Read the model definition and answer for the solid it produces. Units are mm, in the model's axes. Face numbers are marked on the shaded views. A direction names the side the tool comes from. Coordinates: 2 decimals unless noted, no trailing zeros. Write each loop counter-clockwise with the first axis right and the second up, starting at its lowest first coordinate (ties: lowest second). Pieces come first, ordered by that corner, then holes.
(1) Determine the mould class of the marked faces 3, 4 and 5 for opening direction Y: pulls with the +Y half, pulls with the -Y half, needs draft (parallel to the pull), parting line crosses it, or undercut.
(2) The part is cut by section A-A, the plane z = -10. Determine the outline of the cut face in (x, y), and give its area (3 significant figures).
(3) The part is cut by section D-D, the plane z = 0. Determine the outline of the cut face in (x, y), and give its area (3 significant figures).
(4) The part is cut by section B-B, the plane y = 0. Determine the outline of the cut face in (x, z).
(5) The part is cut by section C-C, the plane x = 0. Determine the outline of the cut face in (y, z).
(6) Straight lines are drawn through the part: line 1 along X through (y, z) = (-16.5, 2); line 2 along Z through (x, y) = (-2, -8); line 3 along Y through (x, z) = (-24, 0). For each, find the intervals that lie inside material, in ascending order.
(7) Given pin 1 (24 mm diameter, centred on x = -2, y = 2, fed in from +Z); pin 2 (1.8 mm diameter, centred on x = 17.5, y = -6.5, fed in from +Z), each flat-ended and moving along its own axis, determine where each tip first touches the part or whether it passes through.
(8) Which of the six approach directions +Z, -Z, +X, -X, +Y, -Y give full straight-line access (tool end or side, diameter ignored) to the marked faces 1 and 2?
```python
from build123d import *

# Parameters (mm, degrees)
SKETCH1_R           = 7.5
BOSS_EXTRUDE1_DEPTH = 29
CUT_EXTRUDE1_DEPTH  = 68.505555327
SKETCH3_R           = 7
CUT_EXTRUDE2_DEPTH  = 85.917607126
CUT_EXTRUDE3_DEPTH  = 68.505555438


with BuildPart() as part:
    # Sketch1 → Boss-Extrude1 (new, symmetric)
    with BuildSketch(Plane(origin=(0, 0, 0), x_dir=(0, 0, -1), z_dir=(1, 0, 0))):
        with BuildLine():
            Line((-31, 5), (-31, -19))
            Line((-31, -19), (31, -19))
            Line((31, -19), (46, -10.339745962))
            Line((46, -10.339745962), (46, 12.339745962))
            Line((46, 12.339745962), (31, 21))
            Line((31, 21), (5.66060556, 21))
            ThreePointArc((5.66060556, 21), (-14.33939444, 16.82575695), (-31, 5))
        make_face()
        with Locations(Location((0, 0, 0), (0, 0, 180))):
            Circle(SKETCH1_R, mode=Mode.SUBTRACT)
    extrude(amount=BOSS_EXTRUDE1_DEPTH, both=True)

    # Sketch2 → Cut-Extrude1 (cut, through all)
    with BuildSketch(Plane(origin=(0, 21, 0), x_dir=(1, 0, 0), z_dir=(0, 1, 0))):
        Polygon((-29, 31), (-14, 46), (-29, 46), align=None)
        Polygon((29, 31), (29, 46), (14, 46), align=None)
    extrude(amount=-CUT_EXTRUDE1_DEPTH, mode=Mode.SUBTRACT)

    # Sketch3 → Cut-Extrude2 (cut, through all)
    with BuildSketch(Plane(origin=(0, 0, -46), x_dir=(-1, 0, 0), z_dir=(0, 0, -1))):
        with Locations(Location((0, 0, 0), (0, 0, 90))):
            Circle(SKETCH3_R)
    extrude(amount=-CUT_EXTRUDE2_DEPTH, mode=Mode.SUBTRACT)

    # Sketch4 → Cut-Extrude3 (cut, through all)
    with BuildSketch(Plane(origin=(0, 21, 0), x_dir=(1, 0, 0), z_dir=(0, 1, 0))):
        Polygon((-21, -31), (21, -31), (21, -15), (15, -15), (15, 20), (-15, 20), (-15, -15), (-21, -15), align=None)
    extrude(amount=-CUT_EXTRUDE3_DEPTH, mode=Mode.SUBTRACT)


solid = part.part
```
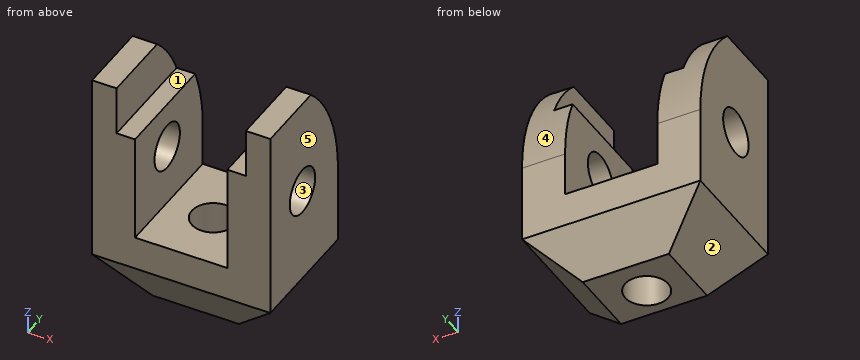
Computed:
1. face 3: undercut
1. face 4: pulls with the +Y half
1. face 5: needs draft
2. outline: (-29, -19) - (-15, -19) - (-15, 21) - (-29, 21) - close; (15, -19) - (29, -19) - (29, 21) - (15, 21) - close
2. area: 1,120 mm2
3. outline: (-29, -19) - (-15, -19) - (-15, -7.5) - (-29, -7.5) - close; (-29, 7.5) - (-15, 7.5) - (-15, 20.68) - (-29, 20.68) - close; (15, -19) - (29, -19) - (29, -7.5) - (15, -7.5) - close; (15, 7.5) - (29, 7.5) - (29, 20.68) - (15, 20.68) - close
3. area: 691 mm2
4. outline: (-29, -31) - (-14, -46) - (-7, -46) - (-7, -20) - (-15, -20) - (-15, -7.5) - (-29, -7.5) - close; (-29, 7.5) - (-15, 7.5) - (-15, 15) - (-21, 15) - (-21, 31) - (-29, 31) - close; (7, -46) - (14, -46) - (29, -31) - (29, -7.5) - (15, -7.5) - (15, -20) - (7, -20) - close; (15, 7.5) - (29, 7.5) - (29, 31) - (21, 31) - (21, 15) - (15, 15) - close
5. outline: (-19, -31) - (-10.34, -46) - (-7, -46) - (-7, -20) - (-19, -20) - close; (7, -46) - (12.34, -46) - (21, -31) - (21, -20) - (7, -20) - close
6. line 1: x = -29 to -15, 15 to 29
6. line 2: z = -46 to -20
6. line 3: y = -19 to -7.5, 7.5 to 20.68
7. pin 1: stops at z = -20
7. pin 2: stops at z = 15
8. face 1: +Z, +Y, -Y
8. face 2: -Z, -X, +Y, -Y
